CAD build for the part. Positions are in the model's coordinates, mm. Coordinates: 2 decimals unless noted, no trailing zeros. Order: outer loops, then holes, each group sorted by start corner. A loop starts at its lowest first (then second) coordinate and runs counter-clockwise, first axis right, second up. Notation, with made-up numbers: (30, -36.75) - (76, -36.75) arc R15 ccw to (76, -19.75) - close; hole circle Ø1 at (-30, 66.5). An arc over 180 degrees is marked (long way). Use one line per item in the form item = value.
```python
from build123d import *

# Parameters (mm, degrees)
F0_W     = 168.927521
F0_H     = 135.896556
F3_DEPTH = 25


with BuildPart() as f2:
    # F0 (on Top) → F2 (revolve)
    with BuildSketch(Plane.XY):
        with Locations((158.588707, 128.150675)):
            Rectangle(F0_W, F0_H)
    revolve(axis=Axis((158.588707, 60.202397, 0), (1, 0, 0)))

    # F1 (on Top) → F3 (join)
    with BuildSketch(Plane.XY):
        Polygon((0, 235.938281), (-136.531189, 235.938281), (-136.531189, -213.123232), (0, -213.123232), (226.407066, 0), align=None)
    extrude(amount=F3_DEPTH)


solid = f2.part
```
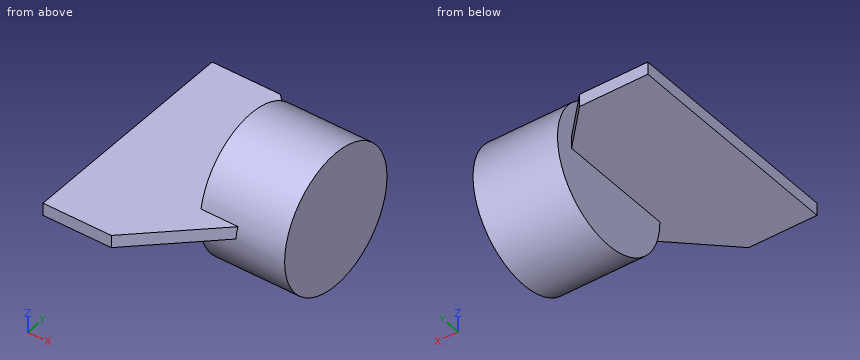
Item 1: Cut at A-A, the plane y = 39. Write the cut outline in (x, z).
Derived:
outline = (-136.53, 0) - (74.12, 0) - (74.12, -134.23) - (243.05, -134.23) - (243.05, 134.23) - (74.12, 134.23) - (74.12, 25) - (-136.53, 25) - close
Item 2: Cut at D-D, the plane x = -77. Write the cut outline in (y, z).
Derived:
outline = (-213.12, 0) - (235.94, 0) - (235.94, 25) - (-213.12, 25) - close
Item 3: Drop flat-ended pins along their axis: pin 1 (4 mm diameter, centred on y = -48.5, z = -11, fed in from -X); pin 2 (1.5 mm diameter, centred on x = -75, y = -79, fed in from -Z); pin 3 (1 mm diameter, centred on x = 128.5, y = -39, fed in from +Z). Give the stop position or say it passes through.
Derived:
pin_1 = 74.12
pin_2 = 0
pin_3 = 93.41
Item 4: Drill centre lines: line 1 (X direction, y = -11, z = 95.5); line 2 (Z direction, x = -61, y = 131.5); line 3 (Y direction, x = 130, z = -2.5). Where is each one in solid material? Low to high. Write a range as [from, to].
Derived:
line_1 = [74.12, 243.05]
line_2 = [0, 25]
line_3 = [-75.67, 196.08]
Item 5: Cut at C-C, the plane z = 13.5. Write the cut outline in (x, y), plus the area to 3 significant figures.
Derived:
outline = (-136.53, -213.12) - (0, -213.12) - (146.71, -75.02) - (243.05, -75.02) - (243.05, 195.43) - (74.12, 195.43) - (74.12, 158.69) - (0, 235.94) - (-136.53, 235.94) - close
area = 137,000 mm²
Item 6: Cut at B-B, the plane x = 197.5. Write the cut outline in (y, z).
Derived:
outline = circle Ø271.79 at (60.2, 0)
